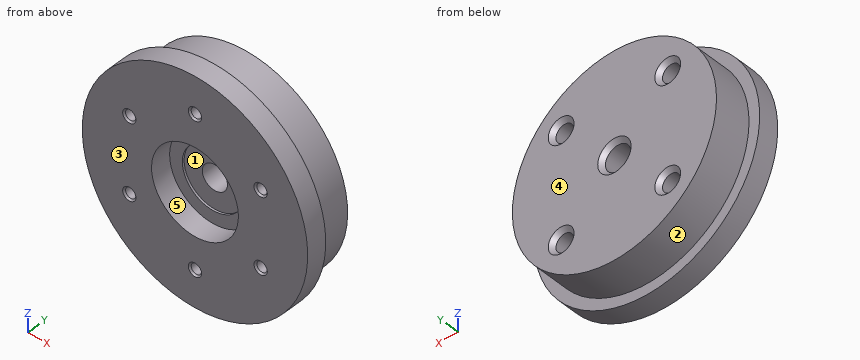
```python
from build123d import *

# Parameters (mm, degrees)
F_2_5_2_5_DURCHMESSER_BOHRUNG1_D           = 2.5
F_2_5_2_5_DURCHMESSER_BOHRUNG1_DEPTH       = 9
F_2_5_2_5_DURCHMESSER_BOHRUNG1_CSINK_D     = 3.25
F_2_5_2_5_DURCHMESSER_BOHRUNG1_CSINK_ANGLE = 90
F_2_5_2_5_DURCHMESSER_BOHRUNG1_TIP         = 0.751075774
SKIZZE5_R                                  = 3.075
SKIZZE5_R_2                                = 2.15
SCHNITT_LINEAR_AUSTRAGEN1_DEPTH            = 9
FASE1_SIZE                                 = 1


with BuildPart() as part:
    # Skizze1 → Rotation1 (revolve)
    with BuildSketch(Plane.XY, mode=Mode.PRIVATE) as rotation1_sk:
        Polygon((10.6, 0), (27.5, 0), (27.5, 5), (24.9, 5), (24.9, 14), (0, 14), (0, 5.5), (7.5, 5.5), (7.5, 5), (10.6, 5), align=None)
    revolve(rotation1_sk.sketch.rotate(Axis((0, 0, 0), (0, -1, 0)), 90), axis=Axis((0, 0, 0), (0, -1, 0)))

    # Ø2.5 (2.5) Durchmesser Bohrung1
    with Locations(Plane(origin=(0, 0, 0), x_dir=(-1, 0, 0), z_dir=(0, -1, 0))):
        with Locations((-16.02146997, 9.25), (0, 18.5), (16.02146997, 9.25), (16.02146997, -9.25), (0, -18.5), (-16.02146997, -9.25)):
            CounterSinkHole(F_2_5_2_5_DURCHMESSER_BOHRUNG1_D / 2, F_2_5_2_5_DURCHMESSER_BOHRUNG1_CSINK_D / 2, depth=F_2_5_2_5_DURCHMESSER_BOHRUNG1_DEPTH, counter_sink_angle=F_2_5_2_5_DURCHMESSER_BOHRUNG1_CSINK_ANGLE)
            with Locations((0, 0, -(F_2_5_2_5_DURCHMESSER_BOHRUNG1_DEPTH + F_2_5_2_5_DURCHMESSER_BOHRUNG1_TIP / 2))):  # 118° drill point
                Cone(0, F_2_5_2_5_DURCHMESSER_BOHRUNG1_D / 2, F_2_5_2_5_DURCHMESSER_BOHRUNG1_TIP, mode=Mode.SUBTRACT)

    # Skizze5 → Schnitt-Linear austragen1 (cut)
    with BuildSketch(Plane(origin=(0, 14, 0), x_dir=(1, 0, 0), z_dir=(0, 1, 0))):
        with Locations(Location((0, 0, 0), (0, 0, 270))):
            Circle(SKIZZE5_R)
        with Locations(Location((13, 13, 0), (0, 0, 270))):
            Circle(SKIZZE5_R_2)
        with Locations(Location((13, -13, 0), (0, 0, 270))):
            Circle(SKIZZE5_R_2)
        with Locations(Location((-13, -13, 0), (0, 0, 270))):
            Circle(SKIZZE5_R_2)
        with Locations(Location((-13, 13, 0), (0, 0, 270))):
            Circle(SKIZZE5_R_2)
    extrude(amount=-SCHNITT_LINEAR_AUSTRAGEN1_DEPTH, mode=Mode.SUBTRACT)

    # Fase1
    fase1_edges = [part.edges().sort_by_distance(p)[0] for p in [
        (-13, 14, -15.15),
        (-13, 14, 10.85),
        (13, 14, 10.85),
        (13, 14, -15.15),
        (0, 14, -3.075),
    ]]
    chamfer(fase1_edges, length=FASE1_SIZE)


solid = part.part
```
Could you check a few things on this model? Use its own coordinates, in mm. Face numbers are marked on the shaded views. A direction names the side the tool comes from. Coordinates: 2 decimals unless noted, no trailing zeros. Write each loop counter-clockwise with the first axis right and the second up, starting at its lowest first coordinate (ties: lowest second). Pieces come first, ordered by that corner, then holes. Notation, with made-up numbers: (54, 1.25) -> (64, 1.25) arc R26 cw to (64, 24.25) -> close; hole circle Ø10 at (42.25, 89). An arc over 180 degrees is marked (long way). Return JSON: item names as keys, results as strings.
(1) I need wall thicknesses on L1, parallel to X at y = 7, z = -9.25; L2, parallel to X at y = 7.5, z = 13; L3, parallel to X at y = 2.5, z = 9.25. Which ranges of each line are inside material? Lowest first, please.
Numbers:
{"L1": "x = -23.12 to -17.27, -14.77 to 14.77, 17.27 to 23.12", "L2": "x = -21.24 to -15.15, -10.85 to 10.85, 15.15 to 21.24", "L3": "x = -25.9 to -17.27, -14.77 to -5.18, 5.18 to 14.77, 17.27 to 25.9"}
(2) Imagine slicing it at C-C, the plane y = 11. Please give me the cut outline in (x, z) (3 decimals), then the cut area to 3 significant figures.
Numbers:
{"outline": "circle Ø49.8 at (0, 0); hole circle Ø4.3 at (-13, -13); hole circle Ø4.3 at (-13, 13); hole circle Ø6.15 at (0, 0); hole circle Ø4.3 at (13, -13); hole circle Ø4.3 at (13, 13)", "area": "1,860 mm2"}
(3) Imagine slicing it at B-B, the plane y = 3.75. Please give me the cut outline in (x, z).
Numbers:
{"outline": "circle Ø55 at (0, 0); hole circle Ø2.5 at (-16.02, -9.25); hole circle Ø2.5 at (-16.02, 9.25); hole circle Ø21.2 at (0, 0); hole circle Ø2.5 at (0, -18.5); hole circle Ø2.5 at (0, 18.5); hole circle Ø2.5 at (16.02, -9.25); hole circle Ø2.5 at (16.02, 9.25)"}
(4) Which directions (+Z, -Z, +X, -X, +Y, -Y) give clear straight access to the entire face, cutting with the end or side of a thin tool? Please do the marked faces 4 and 5.
Numbers:
{"face 4": "+Z, -Z, +X, -X, +Y", "face 5": "-Y"}
(5) I'm going to push flat-ended pins straight in: pin 1 (4.5 mm diameter, centred on x = -14, z = 13.5, fed in from +Y); pin 2 (3.5 mm diameter, centred on x = -13.5, z = -13, fed in from +Y); pin 3 (2 mm diameter, centred on y = 5, z = 20.5, fed in from +X); pin 4 (5 mm diameter, centred on y = 11.5, z = 1.5, fed in from -X). Where does each tip first touch, or does it pass through?
Numbers:
{"pin 1": "stops at y = 14", "pin 2": "stops at y = 13.1", "pin 3": "stops at x = 19.39", "pin 4": "stops at x = -24.9"}
(6) We'd pull the mould along X, two halves only. Please class the marked faces 1, 2 and 3: +X half, -X half, draft (parallel to the pull), parting line (faces both ways), or undercut.
Numbers:
{"face 1": "undercut", "face 2": "parting line", "face 3": "draft"}
(7) Imagine slicing it at A-A, the plane z = 0. Please give me the cut outline in (x, y) (3 decimals), then the cut area to 3 significant figures.
Numbers:
{"outline": "(-27.5, 0) -> (-10.6, 0) -> (-10.6, 5) -> (-7.5, 5) -> (-7.5, 5.5) -> (-3.075, 5.5) -> (-3.075, 13) -> (-4.075, 14) -> (-24.9, 14) -> (-24.9, 5) -> (-27.5, 5) -> close; (3.075, 5.5) -> (7.5, 5.5) -> (7.5, 5) -> (10.6, 5) -> (10.6, 0) -> (27.5, 0) -> (27.5, 5) -> (24.9, 5) -> (24.9, 14) -> (4.075, 14) -> (3.075, 13) -> close", "area": "556 mm2"}
(8) Imagine slicing it at D-D, the plane x = 8.5. Please give me the cut outline in (y, z).
Numbers:
{"outline": "(0, -26.15) -> (5, -26.15) -> (5, -23.4) -> (14, -23.4) -> (14, 23.4) -> (5, 23.4) -> (5, 26.15) -> (0, 26.15) -> (0, 6.33) -> (5, 6.33) -> (5, -6.33) -> (0, -6.33) -> close"}
